Here's the drawing with two shaded views (mm, measured from the low corner). I have some questions. Round coordinates to 2 decimals unless told otherwise and drop trailing zeros. Order: outer loops, then holes, each group sorted by start corner. A loop starts at its lowest first (then second) coordinate and runs counter-clockwise, first axis right, second up.
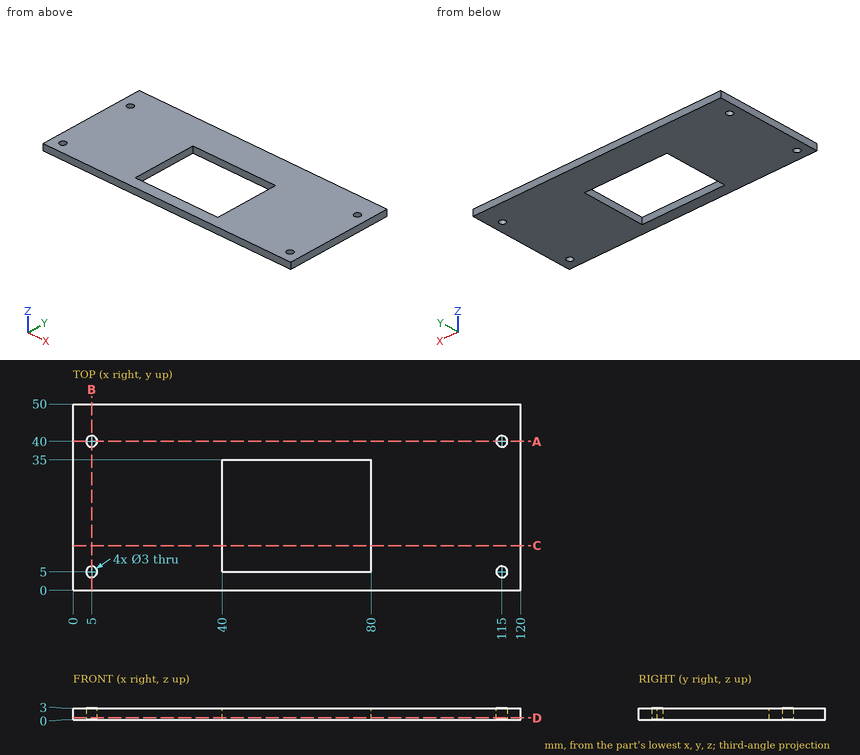
1. If we section it at A-A, the plane y = 40: Write out the boundary of the cut face in (x, z), and give its area (3 significant figures).
Evaluation:
outline: (0, 0) - (3.5, 0) - (3.5, 3) - (0, 3) - close; (6.5, 0) - (113.5, 0) - (113.5, 3) - (6.5, 3) - close; (116.5, 0) - (120, 0) - (120, 3) - (116.5, 3) - close
area: 342 mm2
2. If we section it at B-B, the plane x = 5: Write out the boundary of the cut face in (y, z), and give its area (3 significant figures).
Evaluation:
outline: (0, 0) - (3.5, 0) - (3.5, 3) - (0, 3) - close; (6.5, 0) - (38.5, 0) - (38.5, 3) - (6.5, 3) - close; (41.5, 0) - (50, 0) - (50, 3) - (41.5, 3) - close
area: 132 mm2
3. I need wall thicknesses on probe 1 along Y at (x, z) = (115, 2.05); probe 2 along Y at (x, z) = (50, 1.25); probe 3 along X at (y, z) = (10, 0.9). Which ranges of each line are inside material? Lowest first, please.
Evaluation:
probe 1: y = 0 to 3.5, 6.5 to 38.5, 41.5 to 50
probe 2: y = 0 to 5, 35 to 50
probe 3: x = 0 to 40, 80 to 120
4. If we section it at D-D, the plane z = 0.5: Write out the boundary of the cut face in (x, y).
Evaluation:
outline: (0, 0) - (120, 0) - (120, 50) - (0, 50) - close; hole circle Ø3 at (5, 5); hole circle Ø3 at (5, 40); hole (40, 5) - (80, 5) - (80, 35) - (40, 35) - close; hole circle Ø3 at (115, 5); hole circle Ø3 at (115, 40)
5. I'm going to push flat-ended pins straight in: P1, Ø1.8, axis at x = 5, y = 5, coming from the +Z side; P2, Ø3, axis at x = 33.5, y = 32, coming from the -Z side. Where does each tip first touch, or does it pass through?
Evaluation:
P1: passes through
P2: stops at z = 0
6. If we section it at C-C, the plane y = 12: Write out the boundary of the cut face in (x, z).
Evaluation:
outline: (0, 0) - (40, 0) - (40, 3) - (0, 3) - close; (80, 0) - (120, 0) - (120, 3) - (80, 3) - close
